Geometry: see drawing. Coordinates: mm, zero at the bounding-box minimum. A direction names the side the tool comes from. Give positions to 0.01 mm unless a question says otherwise; leave off trailing zeros. Order: outer loops, then holes, each group sorted by start corner. A loop starts at its lowest first (then second) coordinate and runs counter-clockwise, first axis right, second up. Notation, with made-up numbers: M 81,50 L 88,50 A18 cw 88,61 Z; hole C 85.5,67.5 d7. An arc over 180 degrees is marked long. Return JSON: item names as keys, results as strings.
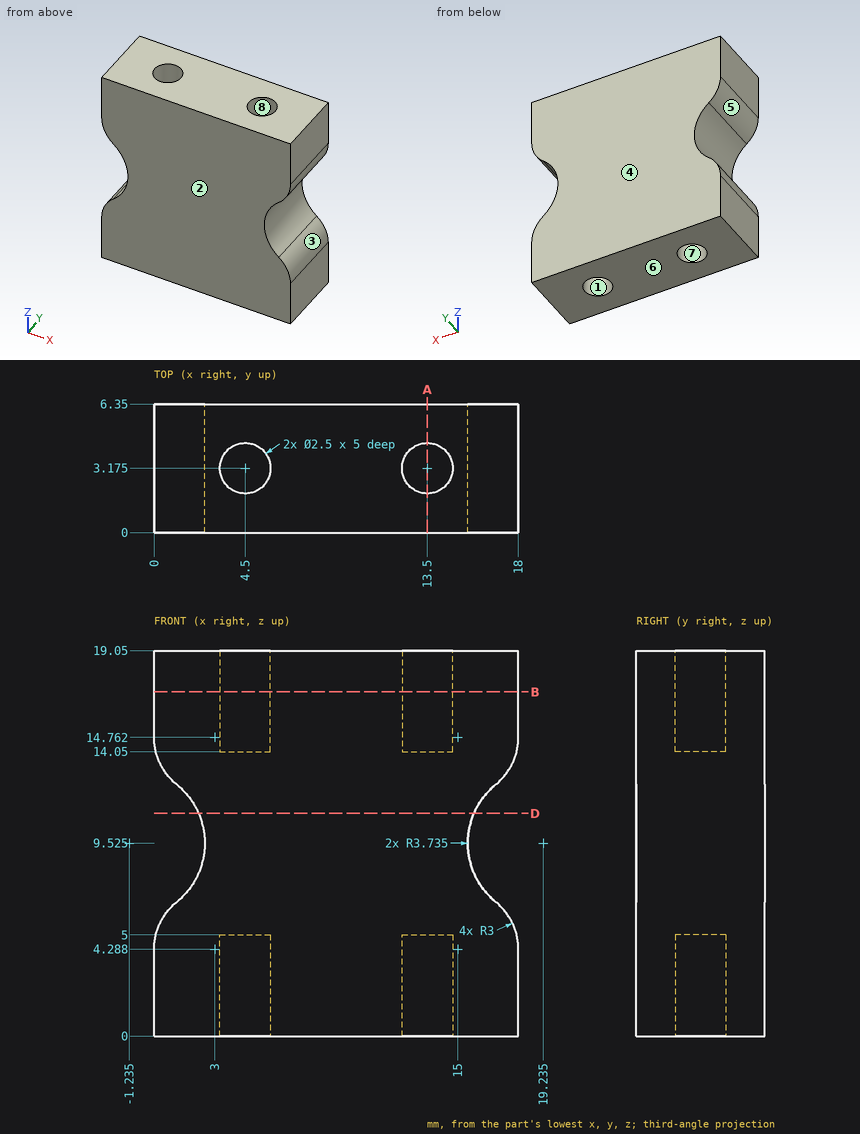
1. Section query A-A (x = 13.5). Return loops of the section in (y, z) (3 decimals).
Evaluation:
{"outline": "M 0,0 L 1.925,0 L 1.925,5 L 4.425,5 L 4.425,0 L 6.35,0 L 6.35,19.05 L 4.425,19.05 L 4.425,14.05 L 1.925,14.05 L 1.925,19.05 L 0,19.05 Z"}
2. Set-up query: the marked faces 4, 5, 6, 7 and 8. Return all of +Z, -Z, +X, -X, +Y, -Y with unobstructed straight access to the full face (end or side cutting, diameter ignored); none if empty.
Evaluation:
{"face 4": "+Z, -Z, +X, -X, +Y", "face 5": "-X, +Y, -Y", "face 6": "-Z, +X, -X, +Y, -Y", "face 7": "-Z", "face 8": "+Z"}
3. Section query D-D (z = 11). Return loops of the section in (x, y).
Evaluation:
{"outline": "M 2.2,0 L 15.8,0 L 15.8,6.35 L 2.2,6.35 Z"}
4. First-contact query: pin 1 (0.8 mm diameter, centred on x = 14, y = 3.5, fed in from +Z); pin 2 (2 mm diameter, centred on x = 4.5, y = 3.175, fed in from -Z). Flat tips, straight axial feed; report the tip coordinate or a pass-through.
Evaluation:
{"pin 1": "stops at z = 14.05", "pin 2": "stops at z = 5"}
5. Draft query along Y for the marked faces 1, 2 and 3. Return one class per face: pulls with the +Y half, pulls with the -Y half, needs draft (parallel to the pull), parting line crosses it, or undercut.
Evaluation:
{"face 1": "undercut", "face 2": "pulls with the -Y half", "face 3": "needs draft"}
6. Ray query, probe 1 along Y at (x, z) = (4.5, 2.2) (3 decimals); probe 2 along X at (y, z) = (4.25, 3.75); probe 3 along Z at (x, y) = (2, 4.25). Return the intervals inside material, ascending.
Evaluation:
{"probe 1": "y = 0 to 1.925, 4.425 to 6.35", "probe 2": "x = 0 to 3.86, 5.14 to 12.86, 14.14 to 18", "probe 3": "z = 0 to 7.66, 11.39 to 19.05"}
7. Section query B-B (z = 17). Return loops of the section in (x, y) (3 decimals), then the cut area to 3 significant figures.
Evaluation:
{"outline": "M 0,0 L 18,0 L 18,6.35 L 0,6.35 Z; hole C 4.5,3.175 d2.5; hole C 13.5,3.175 d2.5", "area": "104 mm^2"}
